Model file for the job. Use its own axes, mm. A direction names the side the tool comes from. Round coordinates to 2 decimals unless told otherwise and drop trailing zeros. Loops run counter-clockwise (first coordinate to the right, second up) from the corner with the lowest first, then second, coordinate; pieces in that order, holes last. Notation, with made-up numbers: (31, 8) -> (84, 8) arc R19 cw to (84, 39) -> close; hole circle Ø7 at (32.5, 13). An arc over 180 degrees is marked (long way). Use a Markdown table: item, result.
from build123d import *

# Parameters (mm, degrees)
PAD035_DEPTH    = 1.85
POCKET020_DEPTH = 6.136478
SKETCH051_W     = 0.3
SKETCH051_H     = 0.7
PAD036_DEPTH    = 0.5
SKETCH052_W     = 0.3
SKETCH052_H     = 0.7
PAD037_DEPTH    = 0.5


with BuildPart() as part:
    # Sketch049 → Pad035 (new body, symmetric)
    with BuildSketch(Plane.XZ):
        with BuildLine():
            Line((-5.3, 5.3), (-5.3, 3.85))
            Line((-5.3, 3.85), (-5, 3.85))
            Line((-5, 3.85), (-5, 5.069802))
            Line((-5, 5.069802), (7.89529, 8.525084))
            Line((8.836014, 9.465809), (7.89529, 8.525084))
            ThreePointArc((10.094687, 9.114411), (9.568018, 9.657855), (8.836014, 9.465809))
            Line((10.094687, 9.114411), (10.38451, 9.192069))
            ThreePointArc((10.38451, 9.192069), (9.645667, 9.947644), (8.623882, 9.677941))
            Line((8.623882, 9.677941), (7.739999, 8.794057))
            Line((-5.3, 5.3), (7.739999, 8.794057))
        make_face()
    extrude(amount=PAD035_DEPTH, both=True)

    # Sketch050 (on Face6 of Pad035) → Pocket020 (cut, through all)
    with BuildSketch(Plane(origin=(0, 0, 3.85), x_dir=(1, 0, 0), z_dir=(0, 0, -1))):
        with BuildLine():
            ThreePointArc((-5.3, 0.35), (-5.65, 0), (-5.3, -0.35))
            Line((-5.3, -0.35), (2.7, -0.35))
            ThreePointArc((2.7, -0.35), (3.05, 0), (2.7, 0.35))
            Line((2.7, 0.35), (-5.3, 0.35))
        make_face()
    extrude(amount=-POCKET020_DEPTH, mode=Mode.SUBTRACT)

    # Sketch051 (on Face5 of Pocket020) → Pad036 (join)
    with BuildSketch(Plane.XZ.offset(1.85)):
        with Locations((-5.15, 4.2)):
            Rectangle(SKETCH051_W, SKETCH051_H)
    extrude(amount=PAD036_DEPTH)

    # Sketch052 (on Face4 of Pad036) → Pad037 (join)
    with BuildSketch(Plane(origin=(0, 1.85, 0), x_dir=(1, 0, 0), z_dir=(0, 1, 0))):
        with Locations((-5.15, -4.2)):
            Rectangle(SKETCH052_W, SKETCH052_H)
    extrude(amount=PAD037_DEPTH)


solid = part.part
Q1. Drill centre lines: L1, parallel to X at y = -0.45, z = 5; L2, parallel to Z at x = 8.25, y = 0.4; L3, parallel to X at y = 0, z = 9. Where is each one in solid material? Low to high. Write a range as from..to.
Results list:
| item | result |
|---|---|
| L1 | x = -5.3..-5 |
| L2 | z = 8.88..9.3 |
| L3 | x = 7.95..8.37 |
Q2. Tool access for faces 1 (the face through (-5.3, 1, 5)), 2 (the face through (8.37, -0.03, 9)), 3 (the face through (-5, 1.3, 4.5)): list every direction of +Z, -Z, +X, -X, +Y, -Y with a clear straight run to the whole face (end or side of a thin tool).
Results list:
| item | result |
|---|---|
| face 1 | +Z, -Z, -X, +Y, -Y |
| face 2 | -Z, +Y, -Y |
| face 3 | -Z, +X, +Y, -Y |
Q3. Band-saw the part on B-B, the plane y = -0.8. Give the cut face in (x, z).
Results list:
| item | result |
|---|---|
| outline | (-5.3, 3.85) -> (-5, 3.85) -> (-5, 5.07) -> (7.9, 8.53) -> (8.84, 9.47) arc R0.75 cw to (10.09, 9.11) -> (10.38, 9.19) arc R1.05 ccw to (8.62, 9.68) -> (7.74, 8.79) -> (-5.3, 5.3) -> close |
Q4. Flat gauge pins, fed straight in: pin 1 (1.1 mm diameter, centred on x = -0.5, z = 6.5, fed in from -Y); pin 2 (1 mm diameter, centred on y = -2, z = 4.5, fed in from +X); pin 3 (1.8 mm diameter, centred on x = -1.5, z = 6, fed in from +Y). Where does each tip first touch, or does it go through?
Results list:
| item | result |
|---|---|
| pin 1 | stops at y = -1.85 |
| pin 2 | stops at x = -5 |
| pin 3 | stops at y = 1.85 |
Q5. Band-saw the part on A-A, the plane z = 4.75. Give the cut face in (x, y), plus the area to 3 significant figures.
Results list:
| item | result |
|---|---|
| outline | (-5.3, -1.85) -> (-5, -1.85) -> (-5, -0.35) -> (-5.3, -0.35) -> close; (-5.3, 0.35) -> (-5, 0.35) -> (-5, 1.85) -> (-5.3, 1.85) -> close |
| area | 0.900 mm² |
Q6. Band-saw the part on C-C, the plane z = 6.75. Give the cut face in (x, y), plus the area to 3 significant figures.
Results list:
| item | result |
|---|---|
| outline | (0.11, -1.85) -> (1.27, -1.85) -> (1.27, -0.35) -> (0.11, -0.35) -> close; (0.11, 0.35) -> (1.27, 0.35) -> (1.27, 1.85) -> (0.11, 1.85) -> close |
| area | 3.48 mm² |
Q7. Band-saw the part on D-D, the plane y = 0. Give the cut face in (x, z).
Results list:
| item | result |
|---|---|
| outline | (3.05, 7.23) -> (7.9, 8.53) -> (8.84, 9.47) arc R0.75 cw to (10.09, 9.11) -> (10.38, 9.19) arc R1.05 ccw to (8.62, 9.68) -> (7.74, 8.79) -> (3.05, 7.54) -> close |
